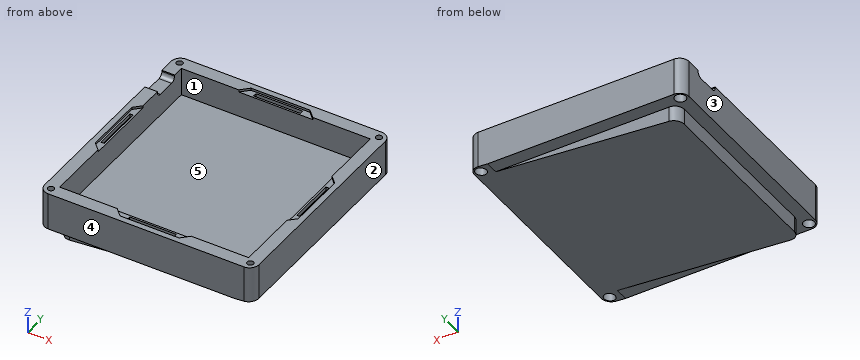
```python
from build123d import *

# Parameters (mm, degrees)
SKETCH1_W                                  = 120.9294
SKETCH1_H                                  = 116.1796
BOSS_EXTRUDE1_DEPTH                        = 5.08
SKETCH2_W                                  = 116.1796
SKETCH2_H                                  = 120.9294
SKETCH2_W_2                                = 102.459137156
SKETCH2_H_2                                = 106.648
BOSS_EXTRUDE2_DEPTH                        = 15.24
CUT_EXTRUDE1_DEPTH                         = 1.25
SKETCH4_W                                  = 25.4
SKETCH4_H                                  = 2.0635
SKETCH4_W_2                                = 1.783031422
SKETCH4_H_2                                = 25.4
CUT_EXTRUDE2_DEPTH                         = 2
CUT_EXTRUDE3_DEPTH                         = 9.906
SKETCH7_R                                  = 3
CUT_EXTRUDE4_DEPTH                         = 12.32
SKETCH8_R                                  = 1.7
CUT_EXTRUDE5_DEPTH                         = 12.32
MIRROR1_AT_THE_SECOND_PLANE_COPY_1_SKETC_R = 3
MIRROR1_AT_THE_SECOND_PLANE_COPY_1_DEPTH   = 12.32
MIRROR1_AT_THE_SECOND_PLANE_COPY_2_SKETC_R = 1.7
MIRROR1_AT_THE_SECOND_PLANE_COPY_2_DEPTH   = 12.32
SKETCH6_W                                  = 109.22
SKETCH6_H                                  = 106.6546
BOSS_EXTRUDE3_DEPTH                        = 9.5504
FILLET1_R                                  = 5.08
FILLET2_R                                  = 5
CUT_EXTRUDE6_DEPTH                         = 18.034
CUT_EXTRUDE6_DEPTH_BACK                    = 130.048


with BuildPart() as part:
    # Sketch1 → Boss-Extrude1 (new body)
    with BuildSketch(Plane(origin=(0, 0, 0), x_dir=(0, 1, 0), z_dir=(0, 0, 1))):
        Rectangle(SKETCH1_W, SKETCH1_H)
    extrude(amount=BOSS_EXTRUDE1_DEPTH)

    # Sketch2 → Boss-Extrude2 (add)
    with BuildSketch(Plane.XY.offset(5.08)):
        Rectangle(SKETCH2_W, SKETCH2_H)
        Rectangle(SKETCH2_W_2, SKETCH2_H_2, mode=Mode.SUBTRACT)
    extrude(amount=BOSS_EXTRUDE2_DEPTH)

    # Sketch3 → Cut-Extrude1 (cut)
    with BuildSketch(Plane.XY.offset(20.32)):
        Polygon((-50.0126, -52.3875), (-21, -52.3875), (-16, -57.3875), (16, -57.3875), (21, -52.3875), (50.0126, -52.3875), (50.0126, -21), (55.0126, -16), (55.0126, 16), (50.0126, 21), (50.0126, 52.3875), (21, 52.3875), (16, 57.3875), (-16, 57.3875), (-21, 52.3875), (-50.0126, 52.3875), (-50.0126, 21), (-55.0126, 16), (-55.0126, -16), (-50.0126, -21), align=None)
    extrude(amount=-CUT_EXTRUDE1_DEPTH, mode=Mode.SUBTRACT)

    # Sketch4 → Cut-Extrude2 (cut)
    with BuildSketch(Plane.XY.offset(19.07)):
        with Locations((0, 55.35575)):
            Rectangle(SKETCH4_W, SKETCH4_H)
        with Locations((0, -55.35575)):
            Rectangle(SKETCH4_W, SKETCH4_H)
        with Locations((-53.121084289, 0)):
            Rectangle(SKETCH4_W_2, SKETCH4_H_2)
        with Locations((53.121084289, 0)):
            Rectangle(SKETCH4_W_2, SKETCH4_H_2)
    extrude(amount=-CUT_EXTRUDE2_DEPTH, mode=Mode.SUBTRACT)

    # Sketch5 → Cut-Extrude3 (cut)
    with BuildSketch(Plane(origin=(-58.0898, 0, 0), x_dir=(0, -1, 0), z_dir=(-1, 0, 0))):
        with BuildLine():
            Line((-44.8211, 26.3172), (-34.9603, 26.3172))
            ThreePointArc((-34.9603, 26.3172), (-33.164248776, 25.573251224), (-32.4203, 23.7772))
            Line((-32.4203, 23.7772), (-32.4203, 19.6822))
            ThreePointArc((-32.4203, 19.6822), (-33.164248776, 17.886148776), (-34.9603, 17.1422))
            Line((-34.9603, 17.1422), (-44.8211, 17.1422))
            ThreePointArc((-44.8211, 17.1422), (-46.617151224, 17.886148776), (-47.3611, 19.6822))
            Line((-47.3611, 19.6822), (-47.3611, 23.7772))
            ThreePointArc((-47.3611, 23.7772), (-46.617151224, 25.573251224), (-44.8211, 26.3172))
        make_face()
    extrude(amount=-CUT_EXTRUDE3_DEPTH, mode=Mode.SUBTRACT)

    # Sketch7 → Cut-Extrude4 (cut)
    with BuildSketch(Plane(origin=(0, 0, 0), x_dir=(1, 0, 0), z_dir=(0, 0, -1))):
        with Locations(Location((-54.0258, 56.4007, 0), (0, 0, 180))):
            Circle(SKETCH7_R)
    cut_extrude4 = extrude(amount=-CUT_EXTRUDE4_DEPTH, mode=Mode.SUBTRACT)

    # Sketch8 → Cut-Extrude5 (cut)
    with BuildSketch(Plane(origin=(0, 0, 12.32), x_dir=(1, 0, 0), z_dir=(0, 0, -1))):
        with Locations(Location((-54.0258, 56.4007, 0), (0, 0, 180))):
            Circle(SKETCH8_R)
    cut_extrude5 = extrude(amount=-CUT_EXTRUDE5_DEPTH, mode=Mode.SUBTRACT)

    # Mirror1: Cut-Extrude4, Cut-Extrude5 across plane
    add(cut_extrude4.mirror(Plane.ZX), mode=Mode.SUBTRACT)
    add(cut_extrude5.mirror(Plane.ZX), mode=Mode.SUBTRACT)

    # Mirror1 at the second plane: Cut-Extrude4, Cut-Extrude5 across plane
    add(cut_extrude4.mirror(Plane(origin=(0, 0, 0), x_dir=(0, 0, 1), z_dir=(1, 0, 0))), mode=Mode.SUBTRACT)
    add(cut_extrude5.mirror(Plane(origin=(0, 0, 0), x_dir=(0, 0, 1), z_dir=(1, 0, 0))), mode=Mode.SUBTRACT)

    # Mirror1 at the second plane copy 1 sketc → Mirror1 at the second plane copy 1 (cut)
    with BuildSketch(Plane(origin=(0, 0, 0), x_dir=(-1, 0, 0), z_dir=(0, 0, -1))):
        with Locations(Location((-54.0258, 56.4007, 0), (0, 0, 180))):
            Circle(MIRROR1_AT_THE_SECOND_PLANE_COPY_1_SKETC_R)
    extrude(amount=-MIRROR1_AT_THE_SECOND_PLANE_COPY_1_DEPTH, mode=Mode.SUBTRACT)

    # Mirror1 at the second plane copy 2 sketc → Mirror1 at the second plane copy 2 (cut)
    with BuildSketch(Plane(origin=(0, 0, 12.32), x_dir=(-1, 0, 0), z_dir=(0, 0, -1))):
        with Locations(Location((-54.0258, 56.4007, 0), (0, 0, 180))):
            Circle(MIRROR1_AT_THE_SECOND_PLANE_COPY_2_SKETC_R)
    extrude(amount=-MIRROR1_AT_THE_SECOND_PLANE_COPY_2_DEPTH, mode=Mode.SUBTRACT)

    # Sketch6 → Boss-Extrude3 (add)
    with BuildSketch(Plane(origin=(0, 0, 0), x_dir=(1, 0, 0), z_dir=(0, 0, -1))):
        with Locations((3.4798, 0)):
            Rectangle(SKETCH6_W, SKETCH6_H)
    extrude(amount=BOSS_EXTRUDE3_DEPTH)

    # Fillet1
    fillet1_edges = [part.edges().sort_by_distance(p)[0] for p in [
        (-51.1302, -53.3273, -4.7752),
        (-51.1302, 53.3273, -4.7752),
    ]]
    fillet(fillet1_edges, radius=FILLET1_R)

    # Fillet2
    fillet2_edges = [part.edges().sort_by_distance(p)[0] for p in [
        (58.0898, 60.4647, 10.16),
        (58.0898, -60.4647, 10.16),
        (-58.0898, -60.4647, 10.16),
        (-58.0898, 60.4647, 10.16),
    ]]
    fillet(fillet2_edges, radius=FILLET2_R)

    # Sketch10 → Cut-Extrude6 (cut, two sides: drawn at the far end of the back side and taken through both)
    with BuildSketch(Plane(origin=(0, 53.3273, 0), x_dir=(-1, 0, 0), z_dir=(0, 1, 0)).offset(-CUT_EXTRUDE6_DEPTH_BACK)):
        Polygon((-58.0898, 0.888884821), (51.1302, -8.666627009), (51.1302, -9.5504), (-58.0898, -9.5504), align=None)
    extrude(amount=CUT_EXTRUDE6_DEPTH + CUT_EXTRUDE6_DEPTH_BACK, mode=Mode.SUBTRACT)


solid = part.part
```
Could you check a few things on this model? Use its own coordinates, in mm. Face numbers are marked on the shaded views. A direction names the side the tool comes from. Coordinates: 2 decimals unless noted, no trailing zeros. Loops run counter-clockwise (first coordinate to the right, second up) from the corner with the lowest first, then second, coordinate; pieces in that order, holes last.
1) Will these pins go through, and if not, where does the flat tip stop? pin 1 Ø6 at (x, y) = (27.5, -29.5) entering from +Z; pin 2 Ø4 at (x, y) = (-18.5, 23) entering from -Z; pin 3 Ø1 at (x, y) = (6.5, 12.5) entering from -Z.
Reported:
pin 1: stops at z = 5.08
pin 2: stops at z = -5.99
pin 3: stops at z = -3.67
2) Imagine slicing it at B-B (z = 15.25). List the corners of the cut face in (x, y) for me.
Reported:
outline: (-58.09, -55.46) arc R5 ccw to (-53.09, -60.46) - (53.09, -60.46) arc R5 ccw to (58.09, -55.46) - (58.09, 55.46) arc R5 ccw to (53.09, 60.46) - (-53.09, 60.46) arc R5 ccw to (-58.09, 55.46) - close; hole circle Ø3.4 at (-54.03, -56.4); hole circle Ø3.4 at (-54.03, 56.4); hole (-51.23, -53.32) - (51.23, -53.32) - (51.23, 53.32) - (-51.23, 53.32) - close; hole circle Ø3.4 at (54.03, -56.4); hole circle Ø3.4 at (54.03, 56.4)
3) Which directions (+Z, -Z, +X, -X, +Y, -Y) give clear straight access to the entire face, cutting with the end or side of a thin tool? Please do the marked faces 1 and 2.
Reported:
face 1: +Z
face 2: +Z, -Z, +X, +Y, -Y
4) Imagine slicing it at A-A (y = -42.5). List the corners of the cut face in (x, z) for me, and give its area (3 significant figures).
Reported:
outline: (-58.09, 0) - (-51.13, 0) - (-51.13, -8.67) - (58.09, 0.89) - (58.09, 20.32) - (51.23, 20.32) - (51.23, 5.08) - (-51.23, 5.08) - (-51.23, 20.32) - (-58.09, 20.32) - close
area: 1,220 mm2
5) Thinking about a two-plate mould opening in X: for the marked faces 3, 4 and 5, which applies, released by +X, released by -X, zero draft, split by the parting line, or undercut?
Reported:
face 3: released by -X
face 4: zero draft
face 5: undercut
6) Please list where these lines run through material, in increasing order: line 1 along Y through (x, z) = (42, 9.5); line 2 along X through (y, z) = (23, 10.25); line 3 along X through (y, z) = (56, 18.5).
Reported:
line 1: y = -60.46 to -53.32, 53.32 to 60.46
line 2: x = -58.09 to -51.23, 51.23 to 58.09
line 3: x = -58.06 to -55.68, -52.37 to -12.7, 12.7 to 52.37, 55.68 to 58.06
7) Imagine slicing it at D-D (y = 36.5). List the corners of the cut face in (x, z) for me, and give its area (3 significant figures).
Reported:
outline: (-58.09, 0) - (-51.13, 0) - (-51.13, -8.67) - (58.09, 0.89) - (58.09, 20.32) - (51.23, 20.32) - (51.23, 5.08) - (-51.23, 5.08) - (-51.23, 17.14) - (-58.09, 17.14) - close
area: 1,200 mm2
8) Imagine slicing it at C-C (x = 8.5). List the corners of the cut face in (y, z) for me.
Reported:
outline: (-60.46, 0) - (-53.33, 0) - (-53.33, -3.45) - (53.33, -3.45) - (53.33, 0) - (60.46, 0) - (60.46, 20.32) - (57.39, 20.32) - (57.39, 19.07) - (56.39, 19.07) - (56.39, 17.07) - (54.32, 17.07) - (54.32, 19.07) - (53.32, 19.07) - (53.32, 5.08) - (-53.32, 5.08) - (-53.32, 19.07) - (-54.32, 19.07) - (-54.32, 17.07) - (-56.39, 17.07) - (-56.39, 19.07) - (-57.39, 19.07) - (-57.39, 20.32) - (-60.46, 20.32) - close
